Verification items for the finished model (mm, model axes). Face numbers are marked on the shaded views. A direction names the side the tool comes from. Coordinates: 2 decimals unless noted, no trailing zeros. Order: outer loops, then holes, each group sorted by start corner. A loop starts at its lowest first (then second) coordinate and runs counter-clockwise, first axis right, second up. Notation, with made-up numbers: M 6.25,76.5 L 29.25,76.5 A31 ccw 29.25,100.5 Z; hole C 48.25,79.5 d8. An arc over 180 degrees is marked long. Return JSON: item names as keys, results as strings.
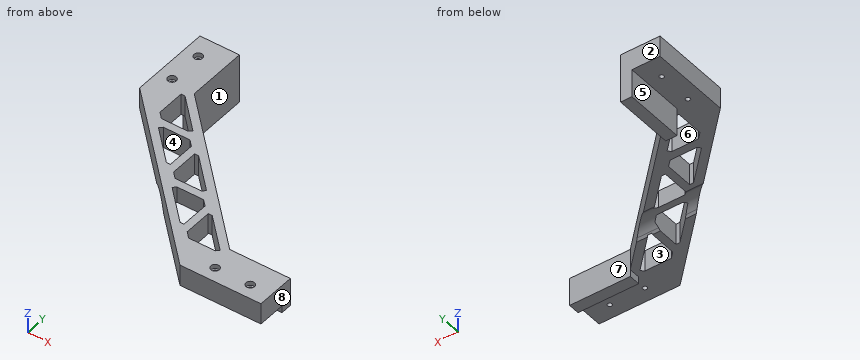
```python
from build123d import *

# Parameters (mm, degrees)
EXTRUDE_1_DEPTH     = 15
SKETCH_3_W          = 43
SKETCH_3_H          = 8
EXTRUDE_2_DEPTH     = 35
SKETCH_4_W          = 8
SKETCH_4_H          = 43
EXTRUDE_3_DEPTH     = 35
CUT_EXTRUDE_1_DEPTH = 244.161454645
SKETCH_6_R          = 1.6
CUT_EXTRUDE_2_DEPTH = 244.161454645
SKETCH_7_R          = 3
CUT_EXTRUDE_3_DEPTH = 3
CHAMFER_1_SIZE      = 2.828427125
CHAMFER_1_SIZE_2    = 4
CUT_EXTRUDE_4_DEPTH = 133
SKETCH_9_W          = 15
SKETCH_9_H          = 8
CUT_EXTRUDE_5_DEPTH = 43


with BuildPart() as part:
    # 草图1 → 凸台-拉伸1 (new body)
    with BuildSketch(Plane.XY):
        Polygon((124.695, -160), (159.695, -160), (159.695, -180), (102.268593129, -180), (-10, -67.731406871), (-10, -10.305), (10, -10.305), (10, -45.305), align=None)
    extrude(amount=EXTRUDE_1_DEPTH)

    # 草图3 → 凸台-拉伸2 (add)
    with BuildSketch(Plane.XY.offset(15)):
        with Locations((138.195, -156)):
            Rectangle(SKETCH_3_W, SKETCH_3_H)
    extrude(amount=-EXTRUDE_2_DEPTH)

    # 草图4 → 凸台-拉伸3 (add)
    with BuildSketch(Plane.XY.offset(15)):
        with Locations((14, -31.805)):
            Rectangle(SKETCH_4_W, SKETCH_4_H)
    extrude(amount=-EXTRUDE_3_DEPTH)

    # 草图5 → 切除-拉伸1 (cut, through all)
    with BuildSketch(Plane.XY.offset(15)):
        Polygon((50.023383861, -93.106558454), (50.023383861, -119.976616139), (76.893441546, -119.976616139), align=None)
        Polygon((55.523383861, -125.476616139), (82.393441546, -125.476616139), (82.393441546, -152.346673824), align=None)
        Polygon((12.153326176, -55.236500769), (12.153326176, -82.106558454), (39.023383861, -82.106558454), align=None)
        Polygon((87.893441546, -130.976616139), (87.893441546, -157.846673824), (114.763499231, -157.846673824), align=None)
        Polygon((17.653326176, -87.606558454), (44.523383861, -87.606558454), (44.523383861, -114.476616139), align=None)
    extrude(amount=-CUT_EXTRUDE_1_DEPTH, mode=Mode.SUBTRACT)

    # 草图6 → 切除-拉伸2 (cut, through all)
    with BuildSketch(Plane.XY.offset(15)):
        with Locations((0, -50.305)):
            Circle(SKETCH_6_R)
        with Locations((0, -25.305)):
            Circle(SKETCH_6_R)
        with Locations((119.695, -170)):
            Circle(SKETCH_6_R)
        with Locations((144.695, -170)):
            Circle(SKETCH_6_R)
    extrude(amount=-CUT_EXTRUDE_2_DEPTH, mode=Mode.SUBTRACT)

    # 草图7 → 切除-拉伸3 (cut)
    with BuildSketch(Plane.XY.offset(15)):
        with Locations((0, -25.305)):
            Circle(SKETCH_7_R)
        with Locations((0, -50.305)):
            Circle(SKETCH_7_R)
        with Locations((119.695, -170)):
            Circle(SKETCH_7_R)
        with Locations((144.695, -170)):
            Circle(SKETCH_7_R)
    extrude(amount=-CUT_EXTRUDE_3_DEPTH, mode=Mode.SUBTRACT)

    # 倒角1
    # the kernel refuses this chamfer: 4, 2.828427125 mm, written as the material it adds along each edge
    with BuildSketch(Plane(origin=(82.393441546, -152.346673824, 15), x_dir=(0.05647824947248942, 0.9984038297885898, 0), z_dir=(0, 0, -1)), Plane(origin=(55.523383861, -125.476616139, 15), x_dir=(0.6660419652145875, -0.7459142715976752, 0), z_dir=(0, 0, -1)), Plane(origin=(87.893441546, -130.976616139, 15), x_dir=(-0.05647824947248942, -0.9984038297885898, 0), z_dir=(0, 0, -1)), Plane(origin=(12.153326176, -55.236500769, 15), x_dir=(-0.05647824947249038, -0.9984038297885897, 0), z_dir=(0, 0, -1)), Plane(origin=(44.523383861, -114.476616139, 15), x_dir=(0.05647824947248914, 0.9984038297885898, 0), z_dir=(0, 0, -1)), Plane(origin=(17.653326176, -87.606558454, 15), x_dir=(0.6660419652145882, -0.7459142715976745, 0), z_dir=(0, 0, -1)), Plane(origin=(50.023383861, -93.106558454, 15), x_dir=(-0.05647824947248914, -0.9984038297885898, 0), z_dir=(0, 0, -1))) as chamfer_1_piece_1:
        Polygon((CHAMFER_1_SIZE * 0.998403829699, -CHAMFER_1_SIZE * 0.0564782494674), (CHAMFER_1_SIZE_2 * 0.666041965215, -CHAMFER_1_SIZE_2 * 0.745914271598), (0, 0), align=None)
    extrude(amount=15)
    with BuildSketch(Plane(origin=(82.393441546, -125.476616139, 15), x_dir=(0.02749587661058555, -0.9996219169112968, 0), z_dir=(0, 0, -1)), Plane(origin=(87.893441546, -157.846673824, 15), x_dir=(-0.02749587661058555, 0.9996219169112968, 0), z_dir=(0, 0, -1)), Plane(origin=(12.153326176, -82.106558454, 15), x_dir=(-0.02749587661058651, 0.9996219169112968, 0), z_dir=(0, 0, -1)), Plane(origin=(44.523383861, -87.606558454, 15), x_dir=(0.027495876610585647, -0.9996219169112968, 0), z_dir=(0, 0, -1)), Plane(origin=(50.023383861, -119.976616139, 15), x_dir=(-0.027495876610585647, 0.9996219169112968, 0), z_dir=(0, 0, -1))) as chamfer_1_piece_2:
        Polygon((CHAMFER_1_SIZE_2 * 0.999621916911, CHAMFER_1_SIZE_2 * 0.0274958766106), (-CHAMFER_1_SIZE_2 * 0.0274958766106, CHAMFER_1_SIZE_2 * 0.999621916911), (0, 0), align=None)
    extrude(amount=15)
    with BuildSketch(Plane(origin=(114.763499231, -157.846673824, 15), x_dir=(-0.9996219169112968, -0.0274958766105891, 0), z_dir=(0, 0, -1)), Plane(origin=(39.023383861, -82.106558454, 15), x_dir=(-0.9996219169112968, -0.027495876610585647, 0), z_dir=(0, 0, -1)), Plane(origin=(76.893441546, -119.976616139, 15), x_dir=(-0.9996219169112968, -0.027495876610585647, 0), z_dir=(0, 0, -1))) as chamfer_1_piece_3:
        Polygon((CHAMFER_1_SIZE_2 * 0.999621916911, CHAMFER_1_SIZE_2 * 0.0274958766106), (CHAMFER_1_SIZE * 0.687396915203, CHAMFER_1_SIZE * 0.726281956812), (0, 0), align=None)
    extrude(amount=15)

    # 草图8 → 切除-拉伸4 (cut)
    with BuildSketch(Plane(origin=(159.695, 0, 0), x_dir=(0, 0, -1), z_dir=(1, 0, 0))):
        with BuildLine():
            Line((-1.18512051, -132.91098195), (0, -134.586598797))
            Line((0, -134.586598797), (0, -115.413471515))
            Line((0, -115.413471515), (-1.18512051, -117.089088362))
            ThreePointArc((-1.18512051, -117.089088362), (-3.7, -125.000035156), (-1.18512051, -132.91098195))
        make_face()
    extrude(amount=-CUT_EXTRUDE_4_DEPTH, mode=Mode.SUBTRACT)

    # 草图9 → 切除-拉伸5 (cut)
    with BuildSketch(Plane(origin=(159.695, 0, 0), x_dir=(0, 0, -1), z_dir=(1, 0, 0))):
        with Locations((12.5, -156)):
            Rectangle(SKETCH_9_W, SKETCH_9_H)
    extrude(amount=-CUT_EXTRUDE_5_DEPTH, mode=Mode.SUBTRACT)


solid = part.part
```
Q1. Cross-section at C-C, the plane z = -16. Record the boundary of the cut face in (x, y) (3 decimals).
Values:
{"outline": "M 10,-53.305 L 18,-53.305 L 18,-10.305 L 10,-10.305 Z"}
Q2. Material ranges on line 1 along X through (y, z) = (-170, 14) (3 decimals); line 2 along Y through (x, z) = (0, 6.5) (3 decimals); line 3 along Y through (x, z) = (0, 13.2) (3 decimals), recorded low to high.
Values:
{"line 1": "92.269 to 116.695, 122.695 to 141.695, 147.695 to 159.695", "line 2": "-77.731 to -51.905, -48.705 to -26.905, -23.705 to -10.305", "line 3": "-77.731 to -53.305, -47.305 to -28.305, -22.305 to -10.305"}
Q3. Cross-section at A-A, the plane y = -100. Record the boundary of the cut face in (x, z) (3 decimals), and give its area (3 significant figures).
Values:
{"outline": "M 22.269,0 L 30.047,0 L 30.047,15 L 22.269,15 Z; M 44.523,0 L 50.023,0 L 50.023,15 L 44.523,15 Z; M 56.917,0 L 64.695,0 L 64.695,15 L 56.917,15 Z", "area": "316 mm^2"}
Q4. Tool access check on the marked faces 5, 6, 7 and 8. Record the directions out of +Z, -Z, +X, -X, +Y, -Y that give a thin tool (end or side, any length) a straight path to the whole face; none if there is none.
Values:
{"face 5": "-Z, -X, +Y, -Y", "face 6": "+Z, -Z", "face 7": "+Z, -Z, +X, +Y", "face 8": "+Z, -Z, +X, +Y, -Y"}
Q5. Cross-section at B-B, the plane x = 125. Record the boundary of the cut face in (y, z).
Values:
{"outline": "M -180,0 L -160,0 L -160,-5 L -152,-5 L -152,15 L -180,15 Z"}
Q6. Cross-section at D-D, the plane z = 7.5. State how many separate pieces and enclosed holes the cut face has, and give its area (3 significant figures).
Values:
{"separate pieces": "1", "enclosed holes": "9", "area": "5,530 mm^2"}
Q7. Go/stop test with flat-tipped pins: pin 1 (12 mm diameter, centred on y = -100.5, z = 8.5, fed in from -X); pin 2 (0.8 mm diameter, centred on x = 13.5, z = 10.5, fed in from -Y); pin 3 (1 mm diameter, centred on y = -32.5, z = 3.5, fed in from +X); pin 4 (1.8 mm diameter, centred on x = 120, y = -170, fed in from +Z). Record where each tip stops, or that it passes through.
Values:
{"pin 1": "x = 16.77", "pin 2": "y = -91.63", "pin 3": "x = 18", "pin 4": "through"}
Q8. Draft check along X on the marked faces 1, 2, 3 and 4. Enter one of: pulls with the +X half, pulls with the -X half, needs draft (parallel to the pull), parting line crosses it, or undercut.
Values:
{"face 1": "pulls with the +X half", "face 2": "needs draft", "face 3": "undercut", "face 4": "undercut"}
